Can you work these out from the model? Positions are in its coordinate system, mm. A direction names the side the tool comes from. Give positions to 0.01 mm unless a question says otherwise; leave off trailing zeros. Loops run counter-clockwise (first coordinate to the right, second up) from the corner with the lowest first, then second, coordinate; pieces in that order, holes last. Notation, with made-up numbers: M 23.25,35.5 L 41.25,35.5 A12 ccw 41.25,45.5 Z; hole C 19,-21.5 d7. An arc over 180 degrees is marked long. One line per item, written item: value. Start each with the question number.
from build123d import *

# Parameters (mm, degrees)
F0_W     = 55
F0_H     = 35
F0_R     = 7.5
F1_DEPTH = 50
F2_T     = -2.5


with BuildPart() as f1:
    # F0 (on Front) → F1 (new body)
    with BuildSketch(Plane.XZ):
        with Locations((27.5, 17.5)):
            Rectangle(F0_W, F0_H)
        with Locations((27.5, 17.5)):
            Circle(F0_R, mode=Mode.SUBTRACT)
    extrude(amount=F1_DEPTH)

    # F2
    f2_openings = [f1.faces().sort_by_distance(p)[0] for p in [
        (27.5, -25, 35),
    ]]
    offset(amount=F2_T, openings=f2_openings)


solid = f1.part
Q1. For P1, Ø6, axis at x = 8.5, y = -32, coming from the +Z side; P2, Ø22.5, axis at x = 21, y = -14, coming from the +Z side, each with a flat end and sliding along its axis, tell me the tip position at first contact or that it passes through.
Q2. If we mould it in two halves opening along Y, with no side actions, what happens to faces 1 (the face through (21, -50, 22)), 2 (the face through (2.5, -25, 19)), 3 (the face through (21.6, -47.5, 26.2)), 4 (the face through (21, 0, 22))? For each: released by +Y, released by -Y, zero draft, split by the parting line, or undercut.
Q3. If we section it at B-B, the plane y = -44.5: Write out the boundary of the cut face in (x, z), plus the area to 3 significant figures.
Q4. I need wall thicknesses on line 1 along X through (y, z) = (-23, 17); line 2 along Z through (x, y) = (27.5, -27.5); line 3 along Y through (x, z) = (48, 29). Which ranges of each line are inside material? Lowest first, please.
Q5. If we section it at D-D, the plane x = 11: Write out the boundary of the cut face in (y, z).
Q6. If we section it at A-A, the plane x = 27.5: Write out the boundary of the cut face in (y, z), plus the area to 4 significant figures.
Q7. If we section it at C-C, the plane z = 17.5: Write out the boundary of the cut face in (x, y).
Q8. Which directions (+Z, -Z, +X, -X, +Y, -Y) give clear straight access to the entire face, cutting with the end or side of a thin tool? Please do faces 5 (the face through (37.04, -24.68, 20.5)), 6 (the face through (52.5, -25, 19)), 7 (the face through (0, -25, 17)).
Response:
1. P1: z = 2.5
1. P2: z = 27.5
2. face 1: released by -Y
2. face 2: undercut
2. face 3: undercut
2. face 4: released by +Y
3. outline: M 0,0 L 55,0 L 55,35 L 52.5,35 L 52.5,2.5 L 2.5,2.5 L 2.5,35 L 0,35 Z; C 27.5,17.5 d20; hole C 27.5,17.5 d15
3. area: 437 mm^2
4. line 1: 0 to 2.5, 17.51 to 20.02, 34.98 to 37.49, 52.5 to 55
4. line 2: 0 to 2.5, 7.5 to 10, 25 to 27.5
4. line 3: -50 to -47.5, -2.5 to 0
5. outline: M -50,0 L 0,0 L 0,35 L -2.5,35 L -2.5,2.5 L -47.5,2.5 L -47.5,35 L -50,35 Z
6. outline: M -50,0 L 0,0 L 0,10 L -50,10 Z; M -50,25 L 0,25 L 0,35 L -2.5,35 L -2.5,27.5 L -47.5,27.5 L -47.5,35 L -50,35 Z; hole M -47.5,2.5 L -2.5,2.5 L -2.5,7.5 L -47.5,7.5 Z
6. area: 437.5 mm^2
7. outline: M 0,-50 L 20,-50 L 20,0 L 0,0 Z; M 35,-50 L 55,-50 L 55,0 L 35,0 Z; hole M 2.5,-47.5 L 17.5,-47.5 L 17.5,-2.5 L 2.5,-2.5 Z; hole M 37.5,-47.5 L 52.5,-47.5 L 52.5,-2.5 L 37.5,-2.5 Z
8. face 5: none
8. face 6: +Z
8. face 7: +Z, -Z, -X, +Y, -Y
